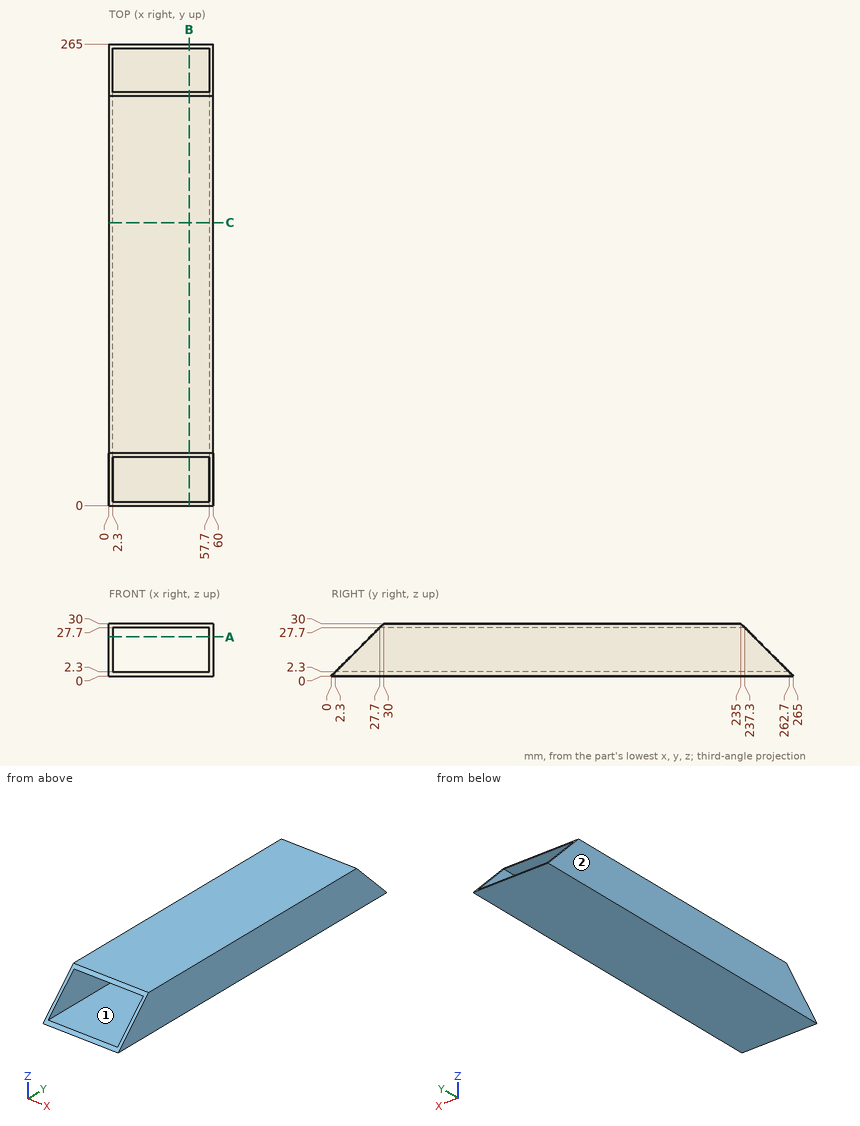
The figure shows three views and two pictorial views of one solid part (mm, origin at its lowest corner). Answer the questions. A direction names the side the tool comes from. Round coordinates to 2 decimals unless told otherwise and drop trailing zeros. Write each loop counter-clockwise with the first axis right and the second up, starting at its lowest first coordinate (ties: lowest second). Pieces come first, ordered by that corner, then holes. Notation, with made-up numbers: (35, -40) - (83, -40) arc R8 ccw to (83, -27) - close; hole circle Ø1 at (32, 17.5). An arc over 180 degrees is marked (long way). One line per question, with ' | ' between items. Start each with the question number.
1. Section B-B (x = 46) is taken. Determine the outline of the cut face in (y, z), and give its area (3 significant figures).
2. Section A-A (z = 22.5) is taken. Determine the outline of the cut face in (x, y).
3. Section C-C (y = 162.5) is taken. Determine the outline of the cut face in (x, z), and give its area (3 significant figures).
4. Find the intervals of material crossed by probe 1 along X at (y, z) = (233.5, 8); probe 2 along Z at (x, y) = (47.5, 156); probe 3 along Z at (x, y) = (51, 249), in increasing order. Write a range as [from, to].
5. This flat-tipped pin is pushed along its axis until it touches: pin 1 (10 mm diameter, centred on x = 49.5, z = 26.5, fed in from -Y). Where does it stop, or does it pass through?
6. For the marked faces 1 and 2, determine the directions among +Z, -Z, +X, -X, +Y, -Y from which every point of the face is accessible in a straight line to the end or side of a thin tool.
Filled in:
1) outline: (0, 0) - (265, 0) - (262.7, 2.3) - (2.3, 2.3) - close; (27.7, 27.7) - (237.3, 27.7) - (235, 30) - (30, 30) - close | area: 1,080 mm²
2) outline: (0, 22.5) - (2.3, 22.5) - (2.3, 242.5) - (0, 242.5) - close; (57.7, 22.5) - (60, 22.5) - (60, 242.5) - (57.7, 242.5) - close
3) outline: (0, 0) - (60, 0) - (60, 30) - (0, 30) - close; hole (2.3, 2.3) - (57.7, 2.3) - (57.7, 27.7) - (2.3, 27.7) - close | area: 393 mm²
4) probe 1: [0, 2.3], [57.7, 60] | probe 2: [0, 2.3], [27.7, 30] | probe 3: [0, 2.3]
5) pin 1: y = 27.7
6) face 1: +Y, -Y | face 2: +Z, -Z, -X, +Y, -Y
